from build123d import *

# Parameters (mm, degrees)
F0_R     = 2.75
F1_DEPTH = 3
F2_R     = 1.5
F3_DEPTH = 18
F4_SIZE  = 0.3
F5_R     = 0.3
F7_DEPTH = 1.5


with BuildPart() as f1:
    # F0 (on Top) → F1 (new body)
    with BuildSketch(Plane.XY):
        Circle(F0_R)
    extrude(amount=F1_DEPTH)

    # F2 (on face) → F3 (join)
    with BuildSketch(Plane(origin=(0, 0, 0), x_dir=(1, 0, 0), z_dir=(0, 0, -1))):
        Circle(F2_R)
    extrude(amount=F3_DEPTH)

    # F4
    f4_edges = [f1.edges().sort_by_distance(p)[0] for p in [
        (-1.5, 0, -18),
    ]]
    chamfer(f4_edges, length=F4_SIZE)

    # F5
    f5_edges = [f1.edges().sort_by_distance(p)[0] for p in [
        (-2.75, 0, 3),
    ]]
    fillet(f5_edges, radius=F5_R)

    # F6 (on face) → F7 (cut)
    with BuildSketch(Plane.XY.offset(3)):
        Polygon((0.721688, 1.25), (-0.721688, 1.25), (-1.443376, 0), (-0.721688, -1.25), (0.721688, -1.25), (1.443376, 0), align=None)
    extrude(amount=-F7_DEPTH, mode=Mode.SUBTRACT)


solid = f1.part
Could you check a few things on this model? Use its own coordinates, in mm. A direction names the side the tool comes from. Coordinates: 2 decimals unless noted, no trailing zeros. Order: outer loops, then holes, each group sorted by start corner. A loop starts at its lowest first (then second) coordinate and runs counter-clockwise, first axis right, second up. Notation, with made-up numbers: (-18.5, 7) -> (-9.5, 7) arc R23 ccw to (-9.5, 19) -> close; hole circle Ø5 at (75, 38.5). An arc over 180 degrees is marked (long way). One line per item, written item: value. Start each with the question number.
1) Imagine slicing it at B-B on z = -1. List the corners of the cut face in (x, y) for me, plus the area to 3 significant figures.
2) If I drill on L1, parallel to Z at x = 1.15, y = 2.2; L2, parallel to Y at x = -0.9, z = -9.5; L3, parallel to Y at x = -0.1, z = -0.75, over which ranges is the centre line in solid material (lowest first)? Write a range as [from, to].
3) I'm going to push flat-ended pins straight in: pin 1 (2 mm diameter, centred on y = 2, z = -9, fed in from -X); pin 2 (2 mm diameter, centred on y = -0.5, z = -15, fed in from -X); pin 3 (2 mm diameter, centred on x = 1, z = -16, fed in from -Y). Where does each tip first touch, or does it pass through?
4) We'd pull the mould along X, two halves only. Please class faces 3 (the flat face through (1.088, 0.616, 2.26)), 4 (the cylindrical face through (-1.5, -0.07, -8.73)), 5 (the flat face through (1.2, -1.2, 0)): +X half, -X half, draft (parallel to the pull), parting line (faces both ways), or undercut.
5) Which directions (+Z, -Z, +X, -X, +Y, -Y) give clear straight access to the entire face, cutting with the end or side of a thin tool? Please do faces 1 (the flat face through (1.1, -1.1, 3)), 2 (the flat face through (0, 0, 1.5)).
6) Imagine slicing it at A-A on x = 0. List the corners of the cut face in (y, z) for me, plus the area to 3 significant figures.
Answer list:
1. outline: circle Ø3 at (0, 0)
1. area: 7.07 mm2
2. L1: z = [0, 3]
2. L2: y = [-1.2, 1.2]
2. L3: y = [-1.5, 1.5]
3. pin 1: stops at x = -1.12
3. pin 2: stops at x = -1.5
3. pin 3: stops at y = -1.5
4. face 3: undercut
4. face 4: parting line
4. face 5: draft
5. face 1: +Z, +X, -X, +Y, -Y
5. face 2: +Z
6. outline: (-2.75, 0) -> (-1.5, 0) -> (-1.5, -17.7) -> (-1.2, -18) -> (1.2, -18) -> (1.5, -17.7) -> (1.5, 0) -> (2.75, 0) -> (2.75, 2.7) arc R0.3 ccw to (2.45, 3) -> (1.25, 3) -> (1.25, 1.5) -> (-1.25, 1.5) -> (-1.25, 3) -> (-2.45, 3) arc R0.3 ccw to (-2.75, 2.7) -> close
6. area: 66.6 mm2
